from build123d import *

# Parameters (mm, degrees)
BOSS_EXTRUDE1_DEPTH  = 25
SKETCH2_W            = 22
SKETCH2_H            = 17
CUT_EXTRUDE1_DEPTH   = 10
M4_CLEARANCE_HOLE1_D = 4.5
M6_CLEARANCE_HOLE1_D = 6.6


with BuildPart() as part:
    # Sketch1 → Boss-Extrude1 (new, symmetric)
    with BuildSketch(Plane(origin=(0, 0, 0), x_dir=(0, 0, -1), z_dir=(1, 0, 0))):
        Polygon((0, 0), (16, 0), (16, 30), (32, 30), (32, 31), (15, 31), (15, 1), (0, 1), align=None)
    extrude(amount=BOSS_EXTRUDE1_DEPTH, both=True)

    # Sketch2 → Cut-Extrude1 (cut)
    with BuildSketch(Plane(origin=(0, 31, 0), x_dir=(1, 0, 0), z_dir=(0, 1, 0))):
        with Locations((0, 23.5)):
            Rectangle(SKETCH2_W, SKETCH2_H)
    extrude(amount=-CUT_EXTRUDE1_DEPTH, mode=Mode.SUBTRACT)

    # M4 Clearance Hole1 (through all)
    with Locations(Plane(origin=(0, 31, 0), x_dir=(1, 0, 0), z_dir=(0, 1, 0))):
        with Locations((-15, 28.25), (15, 28.25)):
            Hole(M4_CLEARANCE_HOLE1_D / 2)

    # M6 Clearance Hole1 (through all)
    with Locations(Plane(origin=(0, 1, 0), x_dir=(1, 0, 0), z_dir=(0, 1, 0))):
        with Locations((-15, 7.5), (15, 7.5)):
            Hole(M6_CLEARANCE_HOLE1_D / 2)


solid = part.part
The listing builds one solid part. Answer for the finished solid, in the listing's coordinates (mm). A direction names the side the tool comes from. Round coordinates to 2 decimals unless told otherwise and drop trailing zeros. Order: outer loops, then holes, each group sorted by start corner. A loop starts at its lowest first (then second) coordinate and runs counter-clockwise, first axis right, second up. Notation, with made-up numbers: (64, -18) -> (102, -18) arc R29 ccw to (102, 19) -> close; hole circle Ø6 at (-3, 4.25). An arc over 180 degrees is marked (long way). One line per item, written item: value.
Item 1: Straight lines are drawn through the part: L1, parallel to Z at x = 15, y = 0.6; L2, parallel to Z at x = -15, y = 30.6; L3, parallel to Z at x = 1, y = 8. For each, find the intervals that lie inside material, in ascending order.
Taken from the geometry:
L1: z = -16 to -10.8, -4.2 to 0
L2: z = -32 to -30.5, -26 to -15
L3: z = -16 to -15
Item 2: Find section B-B, the plane y = 23.5. Give the vertices of the cut face in (x, z), then the cut area to 3 significant figures.
Taken from the geometry:
outline: (-25, -16) -> (-11, -16) -> (-11, -15) -> (-25, -15) -> close; (11, -16) -> (25, -16) -> (25, -15) -> (11, -15) -> close
area: 28.0 mm2
Item 3: Find section C-C, the plane x = -15. Give the vertices of the cut face in (y, z).
Taken from the geometry:
outline: (0, -16) -> (30, -16) -> (30, -26) -> (31, -26) -> (31, -15) -> (1, -15) -> (1, -10.8) -> (0, -10.8) -> close; (0, -4.2) -> (1, -4.2) -> (1, 0) -> (0, 0) -> close; (30, -32) -> (31, -32) -> (31, -30.5) -> (30, -30.5) -> close
Item 4: For a pull along Z with two mould halves and no side action, classify faces 1 (the flat face through (0, 11, -16)), 2 (the flat face through (-18, 30, -24)), 3 (the cylindrical face through (13.962, 30.493, -26.254)) as released by +Z, released by -Z, zero draft, split by the parting line, or undercut.
Taken from the geometry:
face 1: released by -Z
face 2: zero draft
face 3: undercut
Item 5: Given P1, Ø11, axis at x = 19.5, z = -20.5, coming from the -Y side; P2, Ø4, axis at x = -16.5, y = 15.5, coming from the +Z side; P3, Ø7, axis at x = -14.5, z = -22, coming from the -Y side; P4, Ø3, axis at x = -1.5, z = -6.5, coming from the +Y side, each flat-ended and moving along its own axis, determine where each tip first touches the part or whether it passes through.
Taken from the geometry:
P1: stops at y = 0
P2: stops at z = -15
P3: stops at y = 30
P4: stops at y = 1
Item 6: For faces 4 (the flat face through (-11, 30.5, -20.3)), 5 (the flat face through (18, 30, -24)), 6 (the flat face through (0, 1, -8)), determine the directions among +Z, -Z, +X, -X, +Y, -Y from which every point of the face is accessible in a straight line to the end or side of a thin tool.
Taken from the geometry:
face 4: +Z, -Z, +Y
face 5: -Z, +X, -X, -Y
face 6: +Z, +X, -X, +Y
Item 7: Find section D-D, the plane z = -20.5. Give the vertices of the cut face in (x, y).
Taken from the geometry:
outline: (-25, 30) -> (-11, 30) -> (-11, 31) -> (-25, 31) -> close; (11, 30) -> (25, 30) -> (25, 31) -> (11, 31) -> close
Item 8: Find section A-A, the plane z = -28.25. Give the vertices of the cut face in (x, y), then the cut area to 3 significant figures.
Taken from the geometry:
outline: (-25, 30) -> (-17.25, 30) -> (-17.25, 31) -> (-25, 31) -> close; (-12.75, 30) -> (-11, 30) -> (-11, 31) -> (-12.75, 31) -> close; (11, 30) -> (12.75, 30) -> (12.75, 31) -> (11, 31) -> close; (17.25, 30) -> (25, 30) -> (25, 31) -> (17.25, 31) -> close
area: 19.0 mm2
